For this review, use the dimensioned drawing (mm, ordinates from the lowest corner) and the shaded views. A direction names the side the tool comes from. Give positions to 0.01 mm unless a question says otherwise; leave off trailing zeros. Write each loop counter-clockwise with the first axis right and the second up, starting at its lowest first coordinate (ties: lowest second). Pieces come first, ordered by that corner, then holes. Notation, with made-up numbers: M -7.5,11 L 38.5,11 A23 ccw 38.5,35 Z; hole C 5,-23.5 d10. An arc over 180 degrees is marked long. One line per item, written item: value. Start each with the question number.
Item 1: To check wall thickness, follow probe 1 along Z at (x, y) = (50, 32); probe 2 along Z at (x, y) = (33, 33); probe 3 along X at (y, z) = (48, 3). State the ranges of each line that lie inside material, in increasing order.
Item 2: Consider section D-D, the plane x = 21. Write out the cut boundary in (y, z).
Item 3: Consider section A-A, the plane z = 20.25. Write out the cut boundary in (x, y).
Item 4: Tool access review of the marked faces 1 and 2: name each direction out of +Z, -Z, +X, -X, +Y, -Y from which nothing blocks a thin tool from reaching the whole face with its end or side.
Item 5: Consider section C-C, the plane y = 24.5. Write out the cut boundary in (x, z).
Item 6: Mouldability with a two-part tool opening along Z and no side actions: class the marked faces 3, 4 and 5 as released by +Z, released by -Z, zero draft, split by the parting line, or undercut.
Item 7: Clearance check with flat-ended pins moving along their axes: pin 1 Ø5 at (y, z) = (47, 14) entering from -X; pin 2 Ø1.5 at (x, z) = (20, 12.5) entering from +Y; pin 3 Ø7 at (x, z) = (50, 20.25) entering from +Y; pin 4 Ø1.5 at (y, z) = (40.5, 3) entering from -X. State where each tip first meets the part, or that it passes through.
Item 8: Consider section B-B, the plane x = 50. Write out the cut boundary in (y, z).
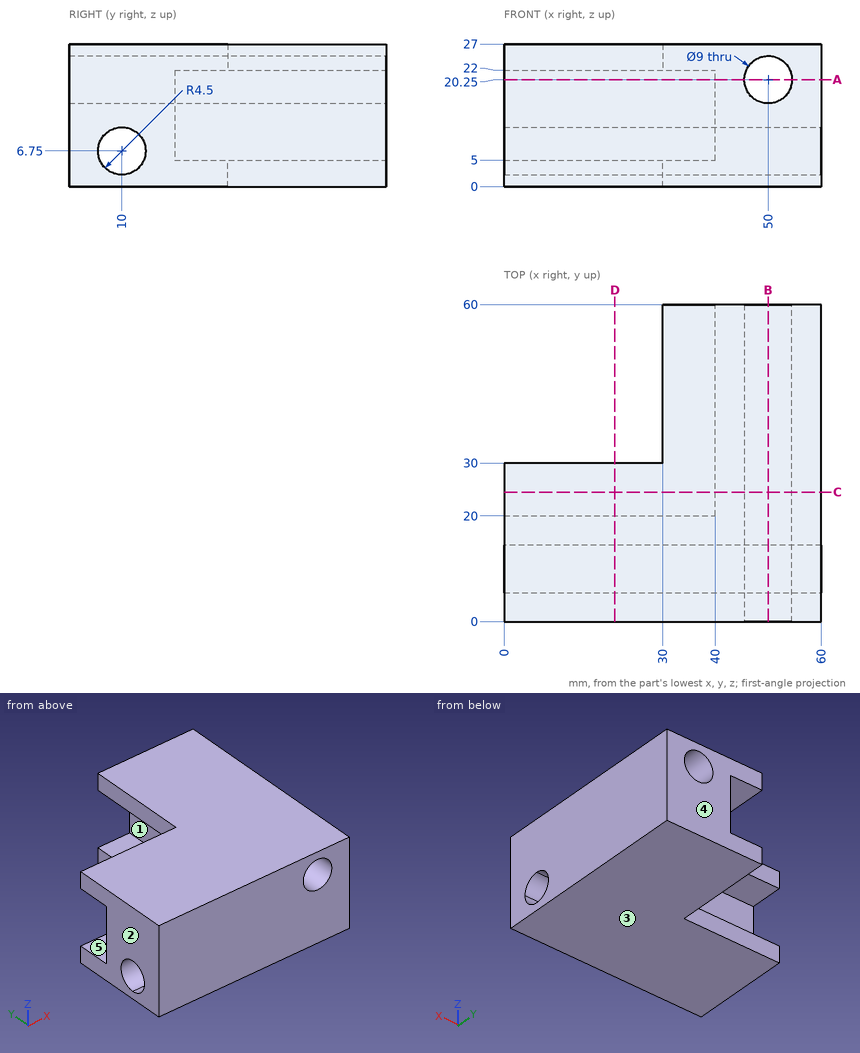
Model answer:
1. probe 1: z = 0 to 15.75, 24.75 to 27
1. probe 2: z = 0 to 5, 22 to 27
1. probe 3: x = 30 to 60
2. outline: M 0,0 L 30,0 L 30,5 L 20,5 L 20,22 L 30,22 L 30,27 L 0,27 Z; hole C 10,6.75 d9
3. outline: M 0,0 L 45.5,0 L 45.5,60 L 40,60 L 40,20 L 0,20 Z; M 54.5,0 L 60,0 L 60,60 L 54.5,60 Z
4. face 1: -X, +Y
4. face 2: +Z, -Z, -X, +Y, -Y
5. outline: M 0,0 L 60,0 L 60,27 L 0,27 L 0,22 L 40,22 L 40,5 L 0,5 Z; hole C 50,20.25 d9
6. face 3: released by -Z
6. face 4: zero draft
6. face 5: undercut
7. pin 1: stops at x = 40
7. pin 2: stops at y = 20
7. pin 3: passes through
7. pin 4: stops at x = 30
8. outline: M 0,0 L 60,0 L 60,15.75 L 0,15.75 Z; M 0,24.75 L 60,24.75 L 60,27 L 0,27 Z; hole C 10,6.75 d9
